The listing builds one solid part. Answer for the finished solid, in the listing's coordinates (mm). Coordinates: 2 decimals unless noted, no trailing zeros. Order: outer loops, then holes, each group sorted by start corner. A loop starts at its lowest first (then second) coordinate and runs counter-clockwise, first axis right, second up. Notation, with made-up numbers: (3.5, 22) -> (22.5, 22) arc R27 cw to (22.5, 48) -> close; hole circle Ø10 at (17.25, 85.5). An arc over 180 degrees is marked (long way). One line per question, with ' | ' between items.
from build123d import *

# Parameters (mm, degrees)
ESQUISSE1_R        = 26.5
ESQUISSE1_R_2      = 3
BOSS_EXTRU_1_DEPTH = 4.5
ESQUISSE2_R        = 12.5
ESQUISSE2_R_2      = 2.8
BOSS_EXTRU_2_DEPTH = 11


with BuildPart() as part:
    # Esquisse1 → Boss.-Extru.1 (new body)
    with BuildSketch(Plane.XY):
        Circle(ESQUISSE1_R)
        Circle(ESQUISSE1_R_2, mode=Mode.SUBTRACT)
    extrude(amount=-BOSS_EXTRU_1_DEPTH)

    # Esquisse2 → Boss.-Extru.2 (add)
    with BuildSketch(Plane.XY):
        Circle(ESQUISSE2_R)
        Circle(ESQUISSE2_R_2, mode=Mode.SUBTRACT)
    extrude(amount=BOSS_EXTRU_2_DEPTH)


solid = part.part
Item 1: Section A-A, the plane x = 0 is taken. Give the vertices of the cut face in (y, z), plus the area to 3 significant figures.
Computed values:
outline: (-26.5, -4.5) -> (-3, -4.5) -> (-3, 0) -> (-2.8, 0) -> (-2.8, 11) -> (-12.5, 11) -> (-12.5, 0) -> (-26.5, 0) -> close; (2.8, 0) -> (3, 0) -> (3, -4.5) -> (26.5, -4.5) -> (26.5, 0) -> (12.5, 0) -> (12.5, 11) -> (2.8, 11) -> close | area: 425 mm^2
Item 2: Section D-D, the plane y = -8.5 is taken. Give the vertices of the cut face in (x, z).
Computed values:
outline: (-25.1, -4.5) -> (25.1, -4.5) -> (25.1, 0) -> (9.17, 0) -> (9.17, 11) -> (-9.17, 11) -> (-9.17, 0) -> (-25.1, 0) -> close
Item 3: Find the intervals of material crossed by L1, parallel to Y at x = 0, z = -2.9; L2, parallel to Y at x = 0, z = 9.25; L3, parallel to Z at x = -19.5, y = 15, in increasing order.
Computed values:
L1: y = -26.5 to -3, 3 to 26.5 | L2: y = -12.5 to -2.8, 2.8 to 12.5 | L3: z = -4.5 to 0
Item 4: Determine the mould class of faces 1 (the face through (-3, 0, -2)), 2 (the face through (11.923, 3.755, 5.423)), 3 (the face through (11.4, -5.5, 0)) for opening direction X: pulls with the +X half, pulls with the -X half, needs draft (parallel to the pull), parting line crosses it, or undercut.
Computed values:
face 1: undercut | face 2: parting line crosses it | face 3: needs draft
Item 5: Each of these flat-tipped pins is pushed along its axis until it touches: pin 1 Ø1.5 at (x, z) = (-16, -1.5) entering from +Y; pin 2 Ø1.5 at (y, z) = (-7, -3) entering from -X; pin 3 Ø6 at (x, z) = (15.5, 0.5) entering from -Y; pin 4 Ø8 at (x, y) = (0, 0) entering from +Z. Where does it stop, or does it pass through?
Computed values:
pin 1: stops at y = 21.67 | pin 2: stops at x = -25.75 | pin 3: stops at y = -23.34 | pin 4: stops at z = 11
Item 6: Section C-C, the plane z = 2 is taken. Give the vertices of the cut face in (x, y).
Computed values:
outline: circle Ø25 at (0, 0); hole circle Ø5.6 at (0, 0)
